For this review, take the finished solid that the model builds, in its own axes (mm). Give positions to 0.01 mm unless a question says otherwise; leave off trailing zeros. Order: outer loops, then holes, each group sorted by start corner. A loop starts at its lowest first (then second) coordinate and runs counter-clockwise, first axis right, second up. Notation, with made-up numbers: M 56,-30 L 114,-30 A34 cw 114,0 Z; hole C 22.25,-20 d7. An arc over 180 degrees is marked long. Use CSV: the item, a comma, the result in double quotes. Start each with the question number.
(1) Clearance check with flat-ended pins moving along their axes: P1, Ø5, axis at x = -64, y = -21, coming from the -Z side; P2, Ø0.9, axis at y = -27, z = 1.5, coming from the -X side. State where each tip first meets the part, or that it passes through.
(2) Consider section A-A (x = -111). Write out the cut boundary in (y, z), and give its area (3 significant figures).
(3) Wall thickness on L1, parallel to Y at x = -130, z = 2.1; L2, parallel to X at y = -30, z = 2.4: over which ranges is each line inside the solid? List them lowest first. Write a range as from..to.
(4) Consider section B-B (y = -27). Write out the cut boundary in (x, z).
Autodesk Inventor part; units mm, degrees
ref_plane "YZ Plane" through (0, 0, 0) normal (1, 0, 0) x (0, 1, 0)
ref_plane "XZ Plane" through (0, 0, 0) normal (0, 1, 0) x (-1, 0, 0)
ref_plane "XY Plane" through (0, 0, 0) normal (0, 0, 1) x (1, 0, 0)
sketch "Sketch1" plane through (0, 0, 0) normal (0, 0, 1) x (1, 0, 0)
  line L0 (-150, 60) -> (150, 60)
  line L1 (150, 60) -> (150, -60)
  line L2 (150, -60) -> (-150, -60)
  line L3 (-150, -60) -> (-150, 60)
  line L4 (-150, 60) -> (150, -60) construction
  line L5 (150, 60) -> (-150, -60) construction
  point P0 (0, 0)
  dimension "d0" = 300
  dimension "d1" = 120
extrude "Extrusion1" add sketch "Sketch1" along normal blind 3
sketch "Sketch2" plane through (0, 0, 3) normal (0, 0, 1) x (1, 0, 0)
  line L0 (-150, -32) -> (-105, -32)
  line L1 (-105, -32) -> (-105, -23)
  line L2 (-105, -23) -> (-150, -23)
  line L3 (-150, -23) -> (-150, -32)
  point P0 (0, 0)
  dimension "d4" = 45
  dimension "d5" = 9
extrude "Extrusion2" cut sketch "Sketch2" against normal up to surface (3 mm away)
properties part number "base_01[1]"
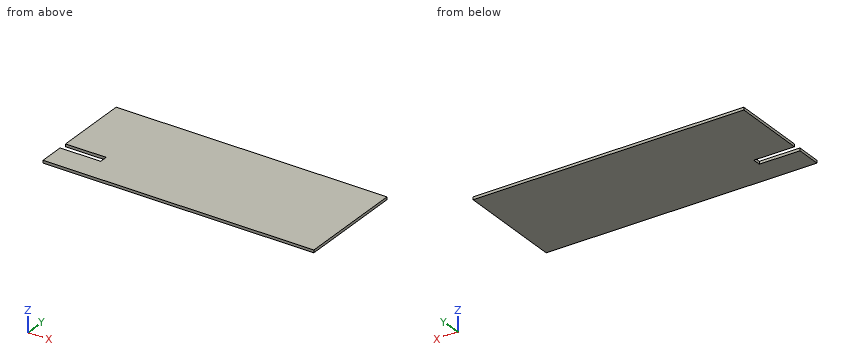
Check result:
1,P1,"stops at z = 0"
1,P2,"stops at x = -105"
2,outline,"M -60,0 L -32,0 L -32,3 L -60,3 Z; M -23,0 L 60,0 L 60,3 L -23,3 Z"
2,area,"333 mm^2"
3,L1,"y = -60..-32, -23..60"
3,L2,"x = -105..150"
4,outline,"M -105,0 L 150,0 L 150,3 L -105,3 Z"
